Geometry check sheet. Reference: drawing and pictorial views, mm from the part's lowest x, y, z. A direction names the side the tool comes from. Round coordinates to 2 decimals unless told otherwise and drop trailing zeros. Write each loop counter-clockwise with the first axis right and the second up, starting at its lowest first coordinate (ties: lowest second). Pieces come first, ordered by that corner, then holes. Notation, with made-up numbers: M -1.75,47.25 L 47.25,47.25 A18 cw 47.25,54.25 Z; hole C -17.5,-39.5 d7. An arc over 180 degrees is marked long. Put each result on its own line as item: value. Start each with the question number.
(1) Section check C-C on y = 42. Record the cut outline in (x, z).
(2) Gauge pin test, flat ends, axial feed: pin 1 (5 mm diameter, centred on x = 6, z = 30.5, fed in from +Y); pin 2 (5 mm diameter, centred on x = 5, y = 20.5, fed in from -Z); pin 3 (8 mm diameter, centred on y = 8, z = 21.5, fed in from +X). Record the tip position at first contact, or that the pin passes through.
(3) Section check D-D on x = 4. Record the cut outline in (y, z).
(4) Tool access check on the marked faces 1 and 2. Record the directions out of +Z, -Z, +X, -X, +Y, -Y that give a thin tool (end or side, any length) a straight path to the whole face; none if there is none.
(5) Section check B-B on z = 27. Record the cut outline in (x, y).
(6) Section check A-A on x = 9.75. Record the cut outline in (y, z).
(7) Material ranges on probe 1 along Y at (x, z) = (11.75, 33); probe 2 along Y at (x, z) = (2, 36), recorded low to high.
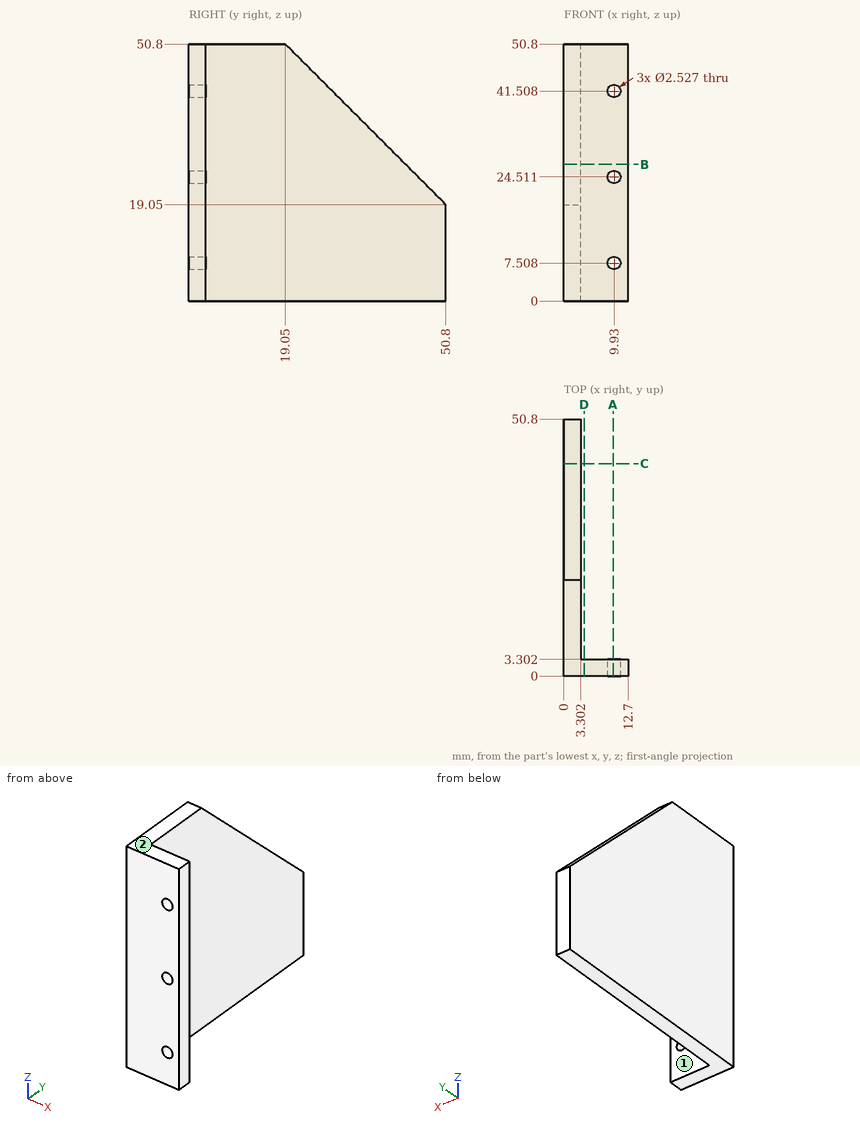
Answers follow:
1. outline: M 0,0 L 3.3,0 L 3.3,27.85 L 0,27.85 Z
2. pin 1: stops at y = 3.3
2. pin 2: stops at z = 0
2. pin 3: stops at x = 3.3
3. outline: M 0,0 L 3.3,0 L 3.3,50.8 L 0,50.8 Z
4. face 1: +Z, -Z, +X, +Y
4. face 2: +Z, +X, -X, +Y, -Y
5. outline: M 0,0 L 12.7,0 L 12.7,3.3 L 3.3,3.3 L 3.3,42.85 L 0,42.85 Z
6. outline: M 0,0 L 3.3,0 L 3.3,6.26 L 0,6.26 Z; M 0,8.76 L 3.3,8.76 L 3.3,23.26 L 0,23.26 Z; M 0,25.76 L 3.3,25.76 L 3.3,40.26 L 0,40.26 Z; M 0,42.76 L 3.3,42.76 L 3.3,50.8 L 0,50.8 Z
7. probe 1: y = 0 to 3.3
7. probe 2: y = 0 to 33.85
